Read the model definition and answer for the solid it produces. Units are mm, in the model's axes. A direction names the side the tool comes from. Round coordinates to 2 decimals unless told otherwise and drop trailing zeros. Order: outer loops, then holes, each group sorted by start corner. A loop starts at its lowest first (then second) coordinate and runs counter-clockwise, first axis right, second up. Notation, with made-up numbers: (-21, 39.25) -> (19, 39.25) arc R13 ccw to (19, 46.25) -> close; hole circle Ø9 at (40, -24). An arc over 180 degrees is marked (long way). One line per item, written item: value. Start each with the question number.
1. The mould has two halves that part along X. Classify faces 4 (the face through (46, 2, -3)), 5 (the face through (2, 2.4, -6.5)), 6 (the face through (46, 4.6, 2)), 7 (the face through (91.1, 2.4, -6.5)): released by +X, released by -X, zero draft, split by the parting line, or undercut.
2. Section A-A (x = 80) is taken. Give the vertices of the cut face in (y, z).
3. A flat-ended cylindrical pin translates along its axis: pin 1 Ø1 at (x, y) = (81, 1.5) entering from +Z. Find the tip coordinate at first contact, or state that the pin passes through.
4. Section B-B (y = 2.25) is taken. Give the vertices of the cut face in (x, z).
5. Consider line 1 (Y direction, x = 54.5, z = -1); line 2 (Z direction, x = 9, y = 1.75); line 3 (Z direction, x = 73, y = 1.75). Determine where each line is inside the solid, lowest interval first.
6. Section D-D (x = 25.5) is taken. Give the vertices of the cut face in (y, z).
7. Section C-C (z = 1.75) is taken. Give the vertices of the cut face in (x, y).
8. For faces 1 (the face through (88.1, 4, -2)), 2 (the face through (85, 2, 0)), 3 (the face through (2, 3.5, -2)), determine the directions among +Z, -Z, +X, -X, +Y, -Y from which every point of the face is accessible in a straight line to the end or side of a thin tool.
from build123d import *

# Parameters (mm, degrees)
SKETCH_2_W                  = 93.1
SKETCH_2_H                  = 10
EXTRUDE_1_DEPTH             = 3.5
SKETCH_4_W                  = 93.1
SKETCH_4_H                  = 6.5
EXTRUDE_2_DEPTH             = 1.1
SKETCH_5_W                  = 93.1
SKETCH_5_H                  = 10
EXTRUDE_3_DEPTH             = 2
CUT_EXTRUDE_1_DEPTH         = 94.867832616
SKETCH_7_W                  = 83.1
SKETCH_7_H                  = 1.1
EXTRUDE_4_DEPTH             = 3.5
CHAMFER_1_SIZE              = 0.4
CUT_EXTRUDE_2_REACH         = 95.868
SKETCH_8_R                  = 150
SKETCH_9_W                  = 93.1
SKETCH_9_H                  = 2
EXTRUDE_5_DEPTH             = 5
EXTRUDE_5_DIRECTION_2_REACH = 95.868
CUT_EXTRUDE_3_REACH         = 95.868
SKETCH_10_W                 = 11.362693304
SKETCH_10_H                 = 0.3
CUT_EXTRUDE_4_REACH         = 95.847
CUT_EXTRUDE_5_REACH         = 95.795


with BuildPart() as part:
    # 草图2 → 凸台-拉伸1 (new body)
    with BuildSketch(Plane(origin=(0, 0, 0), x_dir=(1, 0, 0), z_dir=(0, 1, 0))):
        with Locations((46.55, 5)):
            Rectangle(SKETCH_2_W, SKETCH_2_H)
    extrude(amount=EXTRUDE_1_DEPTH)

    # 草图4 → 凸台-拉伸2 (add)
    with BuildSketch(Plane(origin=(0, 3.5, 0), x_dir=(1, 0, 0), z_dir=(0, 1, 0))):
        with Locations((46.55, 6.75)):
            Rectangle(SKETCH_4_W, SKETCH_4_H)
    extrude(amount=EXTRUDE_2_DEPTH)

    # 草图5 → 凸台-拉伸3 (add)
    with BuildSketch(Plane(origin=(0, 4.6, 0), x_dir=(1, 0, 0), z_dir=(0, 1, 0))):
        with Locations((46.55, 5)):
            Rectangle(SKETCH_5_W, SKETCH_5_H)
    extrude(amount=EXTRUDE_3_DEPTH)

    # 草图6 → 切除-拉伸1 (cut, through all)
    with BuildSketch(Plane.ZY):
        Polygon((-10, 0), (-6.189488223, 6.6), (-10, 6.6), align=None)
    extrude(amount=-CUT_EXTRUDE_1_DEPTH, mode=Mode.SUBTRACT)

    # 草图7 → 凸台-拉伸4 (add)
    with BuildSketch(Plane.XY.offset(-3.5)):
        with Locations((46.55, 4.05)):
            Rectangle(SKETCH_7_W, SKETCH_7_H)
    extrude(amount=EXTRUDE_4_DEPTH)

    # 倒角1
    chamfer_1_edges = [part.edges().sort_by_distance(p)[0] for p in [
        (90.6, 3.5, 0),
        (2.5, 3.5, 0),
    ]]
    chamfer(chamfer_1_edges, length=CHAMFER_1_SIZE)

    # 草图8 → 切除-拉伸2 (cut, up to next)
    with BuildSketch(Plane.XZ, mode=Mode.PRIVATE) as cut_extrude_2_sk1:
        with Locations((46.55, 147)):
            Circle(SKETCH_8_R)
    cut_extrude_2_tool1 = extrude(cut_extrude_2_sk1.sketch, amount=-CUT_EXTRUDE_2_REACH, mode=Mode.PRIVATE) & part.part
    add(cut_extrude_2_tool1.solids().sort_by_distance((46.55, 0, 147))[0], mode=Mode.SUBTRACT)

    # 草图9 → 凸台-拉伸5 (add)
    with BuildSketch(Plane.XY):
        with Locations((46.55, 5.6)):
            Rectangle(SKETCH_9_W, SKETCH_9_H)
    extrude(amount=EXTRUDE_5_DEPTH)

    # 草图9 → 凸台-拉伸5 direction 2 (add, up to next)
    with BuildSketch(Plane.XY, mode=Mode.PRIVATE) as extrude_5_direction_2_sk1:
        with Locations((46.55, 5.6)):
            Rectangle(SKETCH_9_W, SKETCH_9_H)
    extrude_5_direction_2_tool1 = extrude(extrude_5_direction_2_sk1.sketch, amount=-EXTRUDE_5_DIRECTION_2_REACH, mode=Mode.PRIVATE) - part.part
    add(extrude_5_direction_2_tool1.solids().sort_by_distance((46.55, 5.6, 0))[0])

    # 草图10 → 切除-拉伸3 (cut, up to next)
    with BuildSketch(Plane(origin=(93.1, 0, 0), x_dir=(0, 0, -1), z_dir=(1, 0, 0)), mode=Mode.PRIVATE) as cut_extrude_3_sk1:
        with Locations((0.681346652, 6.45)):
            Rectangle(SKETCH_10_W, SKETCH_10_H)
    cut_extrude_3_tool1 = extrude(cut_extrude_3_sk1.sketch, amount=-CUT_EXTRUDE_3_REACH, mode=Mode.PRIVATE) & part.part
    add(cut_extrude_3_tool1.solids().sort_by_distance((93.1, 6.45, -0.681347))[0], mode=Mode.SUBTRACT)

    # 草图11 → 切除-拉伸4 (cut, up to next)
    with BuildSketch(Plane(origin=(93.1, 0, 0), x_dir=(0, 0, -1), z_dir=(1, 0, 0)), mode=Mode.PRIVATE) as cut_extrude_4_sk1:
        Polygon((6.362693304, 6.3), (5.862693304, 6.3), (9.5, 0), (10, 0), align=None)
    cut_extrude_4_tool1 = extrude(cut_extrude_4_sk1.sketch, amount=-CUT_EXTRUDE_4_REACH, mode=Mode.PRIVATE) & part.part
    add(cut_extrude_4_tool1.solids().sort_by_distance((93.1, 3.15, -7.931347))[0], mode=Mode.SUBTRACT)

    # 草图12 → 切除-拉伸5 (cut, up to next)
    with BuildSketch(Plane(origin=(0, 0, 0), x_dir=(1, 0, 0), z_dir=(0, 1, 0)), mode=Mode.PRIVATE) as cut_extrude_5_sk1:
        Polygon((0, 9.5), (5, 9.5), (0, 4.5), align=None)
    cut_extrude_5_tool1 = extrude(cut_extrude_5_sk1.sketch, amount=CUT_EXTRUDE_5_REACH, mode=Mode.PRIVATE) & part.part
    # 草图12 → 切除-拉伸5 (cut, up to next)
    with BuildSketch(Plane(origin=(0, 0, 0), x_dir=(1, 0, 0), z_dir=(0, 1, 0)), mode=Mode.PRIVATE) as cut_extrude_5_sk2:
        Polygon((93.1, 4.5), (93.1, 9.5), (88.1, 9.5), align=None)
    cut_extrude_5_tool2 = extrude(cut_extrude_5_sk2.sketch, amount=CUT_EXTRUDE_5_REACH, mode=Mode.PRIVATE) & part.part
    add(cut_extrude_5_tool1.solids().sort_by_distance((1.666667, 0, -7.833333))[0], mode=Mode.SUBTRACT)
    add(cut_extrude_5_tool2.solids().sort_by_distance((91.433333, 0, -7.833333))[0], mode=Mode.SUBTRACT)


solid = part.part
Answer:
1. face 4: undercut
1. face 5: released by -X
1. face 6: undercut
1. face 7: released by +X
2. outline: (0, -9.5) -> (6.3, -5.86) -> (6.3, 5) -> (4.6, 5) -> (4.6, 0) -> (0, 0) -> close
3. pin 1: z = 0
4. outline: (0, -4.5) -> (3.7, -8.2) -> (89.4, -8.2) -> (93.1, -4.5) -> (93.1, 0) -> (76.4, 0) arc R150 cw to (16.7, 0) -> (0, 0) -> close
5. line 1: 4.6 to 6.3
5. line 2: -8.49 to 0
5. line 3: -8.49 to -0.65
6. outline: (0, -9.5) -> (6.3, -5.86) -> (6.3, 5) -> (4.6, 5) -> (4.6, -1.52) -> (0, -1.52) -> close
7. outline: (0, 4.6) -> (93.1, 4.6) -> (93.1, 6.3) -> (0, 6.3) -> close
8. face 1: +Z, +X
8. face 2: +Z, +X, -X, -Y
8. face 3: +Z, -X
